Autodesk Inventor part; units mm, degrees
ref_plane "Plano de trabalho1" through (-37.5, 6, 11.5) normal (-1, 0, 0) x (0, 0, 1)
ref_plane "YZ Plane" through (0, 0, 0) normal (1, 0, 0) x (0, 1, 0)
ref_plane "XZ Plane" through (0, 0, 0) normal (0, 1, 0) x (-1, 0, 0)
sketch "Esboço1" plane through (0, 0, 0) normal (0, 1, 0) x (-1, 0, 0)
  line L0 (-37.5, 11.5) -> (37.5, 11.5)
  line L1 (37.5, 11.5) -> (37.5, -11.5)
  line L2 (37.5, -11.5) -> (-37.5, -11.5)
  line L3 (-37.5, -11.5) -> (-37.5, 11.5)
  line L4 (-37.5, 11.5) -> (37.5, -11.5) construction
  line L5 (37.5, 11.5) -> (-37.5, -11.5) construction
  point P0 (0, 0)
  dimension "d0" = 75
  dimension "d1" = 23
extrude "Extrusão1" add sketch "Esboço1" along normal blind 18
fillet "Arredondamento1" radius 6 2 edges at (-37.5, 18, 0) (-37.5, 0, 0)
ref_plane "Plano de trabalho1" through (-37.5, 6, 11.5) normal (-1, 0, 0) x (0, 0, 1)
sketch "Esboço2" plane through (-37.5, 6, 11.5) normal (-1, 0, 0) x (0, 0, 1)
  line L0 (-23, -6) -> (-23, 12)
  line L1 (-23, 3) -> (-17.6681, 8.7956) construction
  line L2 (-19.3047, -1.0167) -> (-21.1754, 1.0167) construction
  line L3 (-23, -2.7956) -> (-23, 8.7956)
  line L4 (0, 0) -> (-23, 0)
  circle A0 centre (-20.24, 0) radius 1.3815
  line L5 (-23, 6) -> (0, 6)
  circle A1 centre (-20.24, 6) radius 1.3706
  circle A2 centre (-2.2088, 3) radius 1.0065
  circle A3 centre (-2.2088, 6) radius 1
  circle A4 centre (-2.2088, 0) radius 1
  point P0 (-11.5, -6)
  dimension "d6" = 2
  dimension "d7" = 2
extrude "Extrusão2" add sketch "Esboço2" along normal blind 1.75
fillet "Arredondamento2" radius 2 2 edges at (37.5, 18, 0) (37.5, 0, 0)
fillet "Arredondamento3" radius 1 16 edges at (36.9142, 17.4142, 11.5) (37.5, 9, 11.5) (36.9142, 0.5858, 11.5) (2, 0, 11.5) (-35.7426, 1.7574, 11.5) (-37.5, 9, 11.5) (-35.7426, 16.2426, 11.5) (2, 18, 11.5) (-35.7426, 1.7574, -11.5) (-37.5, 9, -11.5) (-35.7426, 16.2426, -11.5) (2, 18, -11.5) (36.9142, 17.4142, -11.5) (37.5, 9, -11.5) (36.9142, 0.5858, -11.5) (2, 0, -11.5)
sketch "Esboço3" plane through (0, 18, 0) normal (0, 1, 0) x (1, 0, 0)
  line L0 (-29.9595, -10.4813) -> (30.9762, -10.4813) construction
  line L1 (-6.9418, 2.4664) -> (12.8628, 2.4664) construction
  line L2 (12.8628, 2.4664) -> (12.8628, -1.4881) construction
  line L3 (12.8628, -1.4881) -> (-6.9418, -1.4881) construction
  line L4 (-6.9418, -1.4881) -> (-6.9418, 2.4664) construction
  point P0 (0, 0)
properties part number "bateria"
Verification items for the finished model (mm, model axes). A direction names the side the tool comes from. Give positions to 0.01 mm unless a question says otherwise; leave off trailing zeros. Loops run counter-clockwise (first coordinate to the right, second up) from the corner with the lowest first, then second, coordinate; pieces in that order, holes last. Notation, with made-up numbers: M -37.75,75 L 4.25,75 A18 ccw 4.25,94 Z; hole C 68,33 d6. An arc over 180 degrees is marked long. One line per question, with ' | ' between items.
Item 1: Section check B-B, the plane y = 9. Record the cut outline in (x, z), plus the area to 3 significant figures.
Completed:
outline: M -39.25,8.28 L -37.5,8.28 L -37.5,-10.5 A1 ccw -36.5,-11.5 L 36.5,-11.5 A1 ccw 37.5,-10.5 L 37.5,10.5 A1 ccw 36.5,11.5 L -36.5,11.5 A1 ccw -37.5,10.5 L -37.5,10.3 L -39.25,10.3 Z | area: 1,730 mm^2
Item 2: Section check A-A, the plane z = -8.74. Record the cut outline in (x, y).
Completed:
outline: M -39.25,4.62 L -37.5,4.62 L -37.5,6 A6 ccw -31.5,0 L 35.5,0 A2 ccw 37.5,2 L 37.5,16 A2 ccw 35.5,18 L -31.5,18 A6 ccw -37.5,12 L -37.5,13.37 L -39.25,13.37 L -39.25,10.63 L -37.5,10.63 L -37.5,7.38 L -39.25,7.38 Z
Item 3: Thickness scan on line 1 (X direction, y = 10.25, z = -6); line 2 (X direction, y = 16.25, z = 3). Record the ranges inside material, lowest first. Write a range as [from, to].
Completed:
line 1: x = [-37.5, 37.5] | line 2: x = [-35.74, 37.48]
Item 4: Tool access check on faces 1 (the face through (-1, 9, -11.5)), 2 (the face through (-38.36, 9.89, 9.76)). Record the directions out of +Z, -Z, +X, -X, +Y, -Y that give a thin tool (end or side, any length) a straight path to the whole face; none if there is none.
Completed:
face 1: -Z, +X, -X, +Y, -Y | face 2: -X
Item 5: Section check C-C, the plane z = 1.5. Record the cut outline in (x, y).
Completed:
outline: M -37.5,6 A6 ccw -31.5,0 L 35.5,0 A2 ccw 37.5,2 L 37.5,16 A2 ccw 35.5,18 L -31.5,18 A6 ccw -37.5,12 Z
Item 6: Depth check by flat-ended pin: P1, Ø2, axis at y = 15, z = 3.5, coming from the -X side; P2, Ø3, axis at y = 8, z = -2, coming from the -X side. Enter the tip coordinate at first touch or a pass-through.
Completed:
P1: stops at x = -37.16 | P2: stops at x = -37.5
